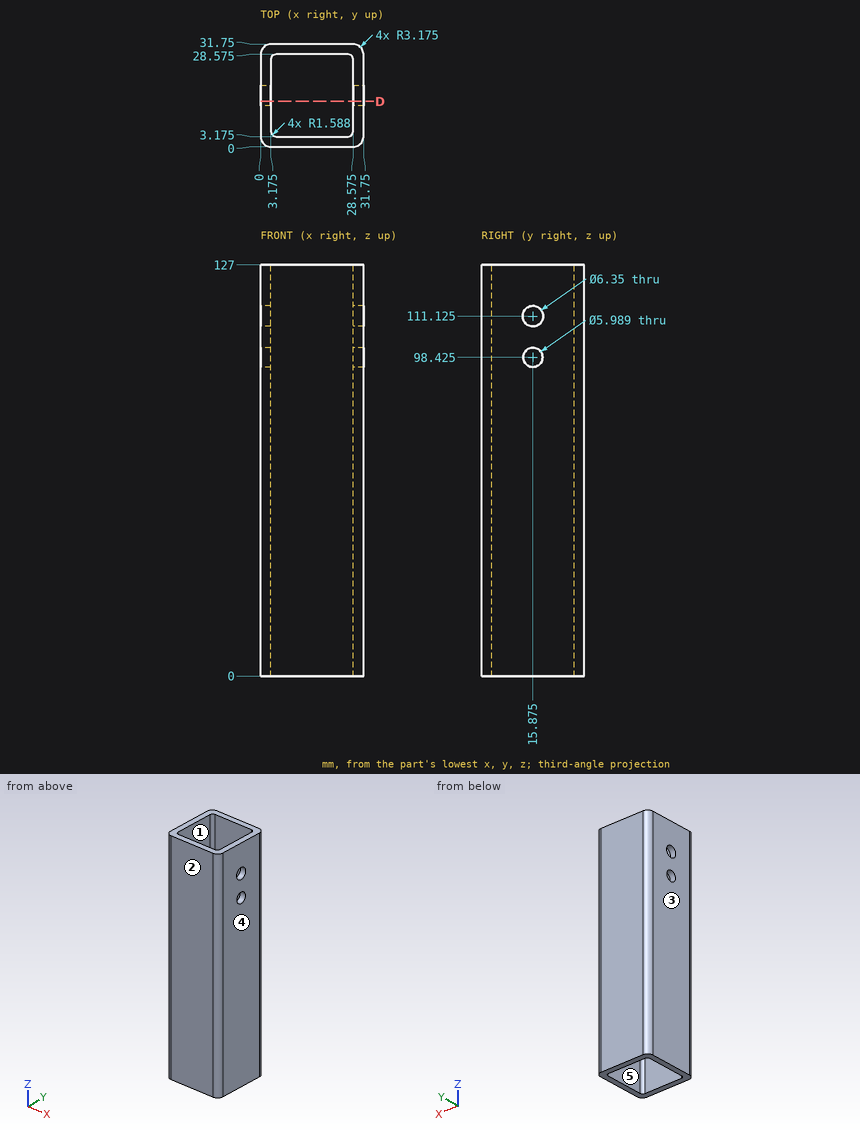
Job drawing, mm, ordinate dimensions from the low corner. One solid piece. A direction names the side the tool comes from. Give positions to 0.01 mm unless a question says otherwise; leave off trailing zeros. Return JSON: item names as keys, results as strings.
Q1. Which spindle directions (+Z, -Z, +X, -X, +Y, -Y) get a long thin tool onto all of the face, cutting with end or side? Do the marked faces 1 and 2. Say none if no direction does.
Working result:
{"face 1": "+Z, -Z", "face 2": "+Z, -Z, +X, -X, -Y"}
Q2. Drill centre line: line 1 (Y direction, x = 30.5, z = 78). Where is it in solid material? Low to high.
Working result:
{"line 1": "0.65 to 31.1"}
Q3. Flat gauge pin, fed straight in: pin 1 (5.5 mm diameter, centred on y = 15.875, z = 98.425, fed in from +X). Where does the tip first touch, or does it go through?
Working result:
{"pin 1": "through"}
Q4. Mould opens along X. For the marked faces 3, 4 and 5 say: pulls with the +X half, pulls with the -X half, needs draft (parallel to the pull), parting line crosses it, or undercut.
Working result:
{"face 3": "pulls with the -X half", "face 4": "pulls with the +X half", "face 5": "undercut"}
Q5. Saw through at D-D (y = 14). Count the separate pieces of the cut face and the enclosed holes in it.
Working result:
{"separate pieces": "6", "enclosed holes": "0"}
